Source: CAD feature listing. Evaluate the final solid. Frame: model axes, mm. A direction names the side the tool comes from. Give positions to 0.01 mm unless a question says otherwise; leave off trailing zeros. Write each loop counter-clockwise with the first axis right and the second up, starting at its lowest first coordinate (ties: lowest second). Pieces come first, ordered by that corner, then holes. Notation, with made-up numbers: (77.25, 24) -> (135.25, 24) arc R28 cw to (135.25, 60) -> close; hole circle Ø6 at (69.25, 80). An arc over 180 degrees is marked (long way). Answer as a JSON object with one key per item and string values. Group by question number.
Item 1: Pull-direction query (X, two-part tool) for faces 3 (the face through (58, -11, 11)), 4 (the face through (-5, -40, 42)), 5 (the face through (25.013, -40.479, 24.428)); classes: pulls with the +X half, pulls with the -X half, needs draft (parallel to the pull), parting line crosses it, or undercut.
Item 2: Section query C-C on x = -24. Return the cut outline in (y, z), plus the area to 3 significant figures.
Item 3: Section query B-B on x = 36.5. Return the cut outline in (y, z).
Item 4: Ray query, probe 1 along Z at (x, y) = (-24, -1); probe 2 along X at (y, z) = (-1, 25); probe 3 along X at (y, z) = (-21, 2). Return the intervals inside material, ascending. Write a range as from..to.
Item 5: Section query A-A on z = 5. Give the number of separate pieces and of enclosed holes in the cut face, plus the area to 3 significant figures.
Item 6: First-contact query: pin 1 Ø6.5 at (x, y) = (-39, -31.5) entering from +Z; pin 2 Ø5.5 at (x, y) = (-40, -33.5) entering from +Z. Flat tips, straight axial feed; report the tip coordinate or a pass-through.
Item 7: Access query for faces 1 (the face through (43.58, -35.59, 4.54)), 2 (the face through (-1, -21, 0)). Directions: +Z, -Z, +X, -X, +Y, -Y. A direction counts if a zero-diameter tool reaches every point of the face in a straight line with its end or side. Return the directions, or none.
from build123d import *

# Parameters (mm, degrees)
SKETCH_W        = 116
SKETCH_H        = 42
PAD_DEPTH       = 42
SKETCH005_W     = 110
SKETCH005_H     = 36
POCKET_DEPTH    = 35
SKETCH006_R     = 1.75
SKETCH006_R_2   = 15
POCKET001_DEPTH = 7.001
POCKET002_DEPTH = 5
SKETCH007_R     = 13
POCKET003_DEPTH = 42.001
SKETCH008_R     = 14
POCKET004_DEPTH = 116.001


with BuildPart() as part:
    # Sketch → Pad (new body)
    with BuildSketch(Plane.XZ):
        with Locations((0, 21)):
            Rectangle(SKETCH_W, SKETCH_H)
    extrude(amount=PAD_DEPTH)

    # Sketch005 → Pocket (cut)
    with BuildSketch(Plane(origin=(0, 0, 42), x_dir=(-1, 0, 0), z_dir=(0, 0, 1))):
        with Locations((0, 21)):
            Rectangle(SKETCH005_W, SKETCH005_H)
    extrude(amount=-POCKET_DEPTH, mode=Mode.SUBTRACT)

    # Sketch006 → Pocket001 (cut, through all)
    with BuildSketch(Plane(origin=(0, 0, 7), x_dir=(-1, 0, 0), z_dir=(0, 0, 1))):
        with Locations((-40, 33.5)):
            Circle(SKETCH006_R)
        with Locations((40, 33.5)):
            Circle(SKETCH006_R)
        with Locations((-40, 9)):
            Circle(SKETCH006_R)
        with Locations((40, 9)):
            Circle(SKETCH006_R)
        with Locations((-20, 21)):
            Circle(SKETCH006_R_2)
        with Locations((20, 21)):
            Circle(SKETCH006_R_2)
    extrude(amount=-POCKET001_DEPTH, mode=Mode.SUBTRACT)

    # Sketch011 → Pocket002 (cut)
    with BuildSketch(Plane(origin=(0, 0, 7), x_dir=(-1, 0, 0), z_dir=(0, 0, 1))):
        Polygon((-42.373287, 37.679591), (-37.615921, 37.679591), (-35.237238, 33.559591), (-37.615921, 29.439591), (-42.373287, 29.439591), (-44.75197, 33.559591), align=None)
        Polygon((37.627177, 37.64135), (42.384544, 37.64135), (44.763227, 33.52135), (42.384544, 29.40135), (37.627177, 29.40135), (35.248494, 33.52135), align=None)
        Polygon((37.575129, 13.14135), (42.332495, 13.14135), (44.711178, 9.02135), (42.332495, 4.90135), (37.575129, 4.90135), (35.196446, 9.02135), align=None)
        Polygon((-42.367844, 13.179591), (-37.610478, 13.179591), (-35.231795, 9.059591), (-37.610478, 4.939591), (-42.367844, 4.939591), (-44.746527, 9.059591), align=None)
    extrude(amount=-POCKET002_DEPTH, mode=Mode.SUBTRACT)

    # Sketch007 → Pocket003 (cut, through all)
    with BuildSketch(Plane(origin=(0, 0, 0), x_dir=(1, 0, 0), z_dir=(0, 1, 0))):
        with Locations((-24, -25)):
            Circle(SKETCH007_R)
        with Locations((7, -25)):
            Circle(SKETCH007_R)
        with Locations((38, -25)):
            Circle(SKETCH007_R)
        with BuildLine():
            ThreePointArc((-43, -16.999991), (-48, -12), (-53, -16.999992))
            Line((-53, -16.999992), (-53, -33.999979))
            ThreePointArc((-53, -33.999979), (-48, -39), (-43, -33.999978))
            Line((-43, -16.999991), (-43, -33.999978))
        make_face()
    extrude(amount=-POCKET003_DEPTH, mode=Mode.SUBTRACT)

    # Sketch008 → Pocket004 (cut, through all)
    with BuildSketch(Plane(origin=(-58, 0, 0), x_dir=(0, 0, -1), z_dir=(-1, 0, 0))):
        with Locations((-23, 22)):
            Circle(SKETCH008_R)
    extrude(amount=-POCKET004_DEPTH, mode=Mode.SUBTRACT)


solid = part.part
Worked answers:
{
 "1": {"face 3": "pulls with the +X half", "face 4": "needs draft", "face 5": "undercut"},
 "2": {"outline": "(-42, 0) -> (-35.46, 0) -> (-35.46, 7) -> (-39, 7) -> (-39, 12) -> (-42, 12) -> close; (-42, 38) -> (-39, 38) -> (-39, 42) -> (-42, 42) -> close; (-6.54, 0) -> (0, 0) -> (0, 12) -> (-3, 12) -> (-3, 7) -> (-6.54, 7) -> close; (-3, 38) -> (0, 38) -> (0, 42) -> (-3, 42) -> close", "area": "146 mm^2"},
 "3": {"outline": "(-42, 0) -> (0, 0) -> (0, 12.09) -> (-3, 12.09) -> (-3, 7) -> (-6.86, 7) -> (-6.86, 2) -> (-11.26, 2) -> (-11.26, 7) -> (-31.37, 7) -> (-31.37, 2) -> (-35.75, 2) -> (-35.75, 7) -> (-39, 7) -> (-39, 12.09) -> (-42, 12.09) -> close; (-42, 37.91) -> (-39, 37.91) -> (-39, 42) -> (-42, 42) -> close; (-3, 37.91) -> (0, 37.91) -> (0, 42) -> (-3, 42) -> close"},
 "4": {"probe 1": "0..12, 38..42", "probe 2": "-58..-53, -43..-37, -11..-6, 20..25, 51..58", "probe 3": "-58..-35, -5..5, 35..58"},
 "5": {"separate pieces": "1", "enclosed holes": "6", "area": "3,220 mm^2"},
 "6": {"pin 1": "z = 7", "pin 2": "z = 2"},
 "7": {"face 1": "+Z", "face 2": "-Z, +X, -X, +Y, -Y"}
}
